Geometry check sheet. Reference: the model listing, model coordinates, mm. A direction names the side the tool comes from. Round coordinates to 2 decimals unless told otherwise and drop trailing zeros. Loops run counter-clockwise (first coordinate to the right, second up) from the corner with the lowest first, then second, coordinate; pieces in that order, holes last. Notation, with made-up numbers: (-8.75, -39.75) - (35.25, -39.75) arc R26 ccw to (35.25, -18.75) - close; hole circle Ø8 at (49, 28). An arc over 180 degrees is marked (long way). Answer as CSV lines item,"result". Start each with the question number.
1) Cross-section at A-A on x = 0.5. Record the boundary of the cut face in (y, z), and give its area (3 significant figures).
2) Depth check by flat-ended pin: P1, Ø4, axis at x = -0.5, y = 34, coming from the +Z side; P2, Ø2.5, axis at x = 0.88, y = 34.12, coming from the -Z side; P3, Ø0.5, axis at x = 0, z = 2, coming from the +Y side; P4, Ø0.8, axis at x = -2, z = 2.5, coming from the -Y side. Enter the tip coordinate at first touch or a pass-through.
3) Cross-section at C-C on y = 16. Record the boundary of the cut face in (x, z) (3 decimals).
4) Access from +Z, -Z, +X, -X, +Y, -Y to the whole of each face (thin tool, end or side, straight path). Record for faces 4 (the flat face through (1, 27.775, 2)), 5 (the flat face through (1, 2.375, 2)), 6 (the cylindrical face through (1.23, 35.72, 0.81)).
5) Cross-section at B-B on z = 0.7. Record the boundary of the cut face in (x, y), and give its area (3 significant figures).
6) Cross-section at D-D on x = -3. Record the boundary of the cut face in (y, z).
7) Thickness scan on line 1 along Y through (x, z) = (0.75, 3); line 2 along Z through (x, y) = (-2.25, 29); line 3 along Y through (x, z) = (0, 2.25). Record the ranges inside material, lowest first.
8) Draft check along X on faces 1 (the flat face through (-3, 15, 0)), 2 (the cylindrical face through (1.316, 18.424, 1.565)), 3 (the flat face through (7.228, 15, 1)). Enter one of: released by +X, released by -X, zero draft, split by the parting line, or undercut.
from build123d import *

# Parameters (mm, degrees)
SKETCH1_W                = 12.7
SKETCH1_H                = 50.8
BOSS_EXTRUDE1_DEPTH      = 3.175
CUT_EXTRUDE1_DEPTH       = 42.237466092
CUT_EXTRUDE1_DEPTH_BACK  = 42.237466092
SKETCH4_W                = 1.524
SKETCH4_H                = 12.7
CUT_EXTRUDE9_START       = 2.374796748
CUT_EXTRUDE9_DEPTH       = 25.4
CUT_EXTRUDE15_DEPTH      = 42.237466092
CUT_EXTRUDE15_DEPTH_BACK = 2.54
SKETCH7_R                = 1.63195
SKETCH7_R_2              = 3.3782


# Read off the part's stored shape, not the designer's step: Cut-Extrude9
with BuildPart() as part:
    # Sketch1 → Boss-Extrude1 (new body)
    with BuildSketch(Plane.XY):
        with Locations((0.877642276, 15.074796748)):
            Rectangle(SKETCH1_W, SKETCH1_H)
    extrude(amount=BOSS_EXTRUDE1_DEPTH)

    # Sketch4 → Cut-Extrude1 (cut, two sides: drawn at the far end of the back side and taken through both)
    with BuildSketch(Plane(origin=(0, 0, 0), x_dir=(0, 0, -1), z_dir=(1, 0, 0)).offset(-CUT_EXTRUDE1_DEPTH_BACK)):
        with Locations((-2.413, 34.124796748)):
            Rectangle(SKETCH4_W, SKETCH4_H)
        with Locations((-2.413, -3.975203252)):
            Rectangle(SKETCH4_W, SKETCH4_H)
    extrude(amount=CUT_EXTRUDE1_DEPTH + CUT_EXTRUDE1_DEPTH_BACK, mode=Mode.SUBTRACT)

    # Cut-Extrude9 outline → Cut-Extrude9 (cut)
    with BuildSketch(Plane(origin=(0, 0, 0), x_dir=(1, 0, 0), z_dir=(0, 1, 0)).offset(CUT_EXTRUDE9_START)):
        with BuildLine():
            ThreePointArc((7.227642276, -2.909267581), (3.616263069, -3.10854445), (5.36e-07, -3.175))
            Line((5.36e-07, -3.175), (7.227642276, -3.175))
            Line((7.227642276, -3.175), (7.227642276, -2.909267581))
        make_face()
        with BuildLine():
            ThreePointArc((5.36e-07, -3.175), (-2.737237313, -3.136930824), (-5.472357724, -3.022752714))
            Line((-5.472357724, -3.022752714), (-5.472357724, -3.175))
            Line((-5.472357724, -3.175), (5.36e-07, -3.175))
        make_face()
    extrude(amount=CUT_EXTRUDE9_DEPTH, mode=Mode.SUBTRACT)

    # Sketch7 → Cut-Extrude15 (cut, two sides: drawn at the far end of the back side and taken through both)
    with BuildSketch(Plane.XY.offset(-CUT_EXTRUDE15_DEPTH_BACK)):
        with Locations(Location((0.877642276, -3.975203252, 0), (0, 0, 180))):
            Circle(SKETCH7_R)
        with Locations(Location((0.877642276, 34.124796748, 0), (0, 0, 180))):
            Circle(SKETCH7_R)
        with Locations(Location((0.877642276, 15.074796748, 0), (0, 0, 105.05794783))):
            Circle(SKETCH7_R_2)
    extrude(amount=CUT_EXTRUDE15_DEPTH + CUT_EXTRUDE15_DEPTH_BACK, mode=Mode.SUBTRACT)


solid = part.part
Answer block:
1,outline,"(-10.33, 0) - (-5.56, 0) - (-5.56, 1.65) - (-10.33, 1.65) - close; (-2.39, 0) - (11.72, 0) - (11.72, 3.17) - (2.37, 3.17) - (2.37, 1.65) - (-2.39, 1.65) - close; (18.43, 0) - (32.54, 0) - (32.54, 1.65) - (27.77, 1.65) - (27.77, 3.17) - (18.43, 3.17) - close; (35.71, 0) - (40.47, 0) - (40.47, 1.65) - (35.71, 1.65) - close"
1,area,"90.8 mm^2"
2,P1,"stops at z = 1.65"
2,P2,"passes through"
2,P3,"stops at y = 27.77"
2,P4,"stops at y = 2.37"
3,outline,"(-5.472, 0) - (-2.371, 0) - (-2.371, 3.146) arc R98.425 ccw to (-5.472, 3.023) - close; (4.127, 0) - (7.228, 0) - (7.228, 2.909) arc R98.425 ccw to (4.127, 3.088) - close"
4,face 4,"+Z, +X, -X, +Y"
4,face 5,"+Z, +X, -X, -Y"
4,face 6,"+Z, -Z"
5,outline,"(-5.47, -10.33) - (7.23, -10.33) - (7.23, 40.47) - (-5.47, 40.47) - close; hole circle Ø6.76 at (0.88, 15.07); hole circle Ø3.26 at (0.88, -3.98); hole circle Ø3.26 at (0.88, 34.12)"
5,area,"593 mm^2"
6,outline,"(-10.33, 0) - (40.47, 0) - (40.47, 1.65) - (27.77, 1.65) - (27.77, 3.13) - (2.37, 3.13) - (2.37, 1.65) - (-10.33, 1.65) - close"
7,line 1,"y = 2.37 to 11.7, 18.45 to 27.77"
7,line 2,"z = 0 to 1.65"
7,line 3,"y = 2.37 to 11.81, 18.34 to 27.77"
8,face 1,"zero draft"
8,face 2,"undercut"
8,face 3,"released by +X"
